Geometry check sheet. Reference: the model listing, model coordinates, mm. Coordinates: 2 decimals unless noted, no trailing zeros. Write each loop counter-clockwise with the first axis right and the second up, starting at its lowest first coordinate (ties: lowest second). Pieces come first, ordered by that corner, then holes. Notation, with made-up numbers: (26, 61) -> (56, 61) arc R15 cw to (56, 65) -> close; hole circle Ø7 at (88, 68). An arc over 180 degrees is marked (long way). Answer as CSV lines item,"result".
```python
from build123d import *

# Parameters (mm, degrees)
SKIZZE1_W                       = 45
SKIZZE1_H                       = 85
AUFSATZ_LINEAR_AUSTRAGEN1_DEPTH = 5
SKIZZE3_W                       = 5
SKIZZE3_H                       = 1.5
SKIZZE3_H_2                     = 1.241942413
SCHNITT_LINEAR_AUSTRAGEN1_DEPTH = 5
SKIZZE4_R                       = 1.6
SCHNITT_LINEAR_AUSTRAGEN2_DEPTH = 5


with BuildPart() as part:
    # Skizze1 → Aufsatz-Linear austragen1 (new body)
    with BuildSketch(Plane.XY):
        with Locations((22.5, 42.5)):
            Rectangle(SKIZZE1_W, SKIZZE1_H)
    extrude(amount=AUFSATZ_LINEAR_AUSTRAGEN1_DEPTH)

    # Skizze3 → Schnitt-Linear austragen1 (cut)
    with BuildSketch(Plane.XY.offset(5)):
        with Locations((12.5, 58.8)):
            Rectangle(SKIZZE3_W, SKIZZE3_H)
        with Locations((32.75, 58.8)):
            Rectangle(SKIZZE3_W, SKIZZE3_H)
        with Locations((19.25, 46.8)):
            Rectangle(SKIZZE3_W, SKIZZE3_H)
        with Locations((12.5, 50.8)):
            Rectangle(SKIZZE3_W, SKIZZE3_H)
        with Locations((32.75, 50.8)):
            Rectangle(SKIZZE3_W, SKIZZE3_H)
        with Locations((12.5, 42.8)):
            Rectangle(SKIZZE3_W, SKIZZE3_H)
        with Locations((32.75, 42.8)):
            Rectangle(SKIZZE3_W, SKIZZE3_H)
        with Locations((12.5, 34.8)):
            Rectangle(SKIZZE3_W, SKIZZE3_H)
        with Locations((32.75, 34.8)):
            Rectangle(SKIZZE3_W, SKIZZE3_H)
        with Locations((32.75, 26.8)):
            Rectangle(SKIZZE3_W, SKIZZE3_H)
        with Locations((12.5, 26.8)):
            Rectangle(SKIZZE3_W, SKIZZE3_H)
        with Locations((19.25, 54.929028794)):
            Rectangle(SKIZZE3_W, SKIZZE3_H_2)
        with Locations((26, 54.929028794)):
            Rectangle(SKIZZE3_W, SKIZZE3_H_2)
        with Locations((26, 46.8)):
            Rectangle(SKIZZE3_W, SKIZZE3_H)
        with Locations((26, 38.8)):
            Rectangle(SKIZZE3_W, SKIZZE3_H)
        with Locations((19.25, 38.8)):
            Rectangle(SKIZZE3_W, SKIZZE3_H)
        with Locations((19.25, 30.8)):
            Rectangle(SKIZZE3_W, SKIZZE3_H)
        with Locations((26, 30.8)):
            Rectangle(SKIZZE3_W, SKIZZE3_H)
        with Locations((26, 22.8)):
            Rectangle(SKIZZE3_W, SKIZZE3_H)
        with Locations((19.25, 22.8)):
            Rectangle(SKIZZE3_W, SKIZZE3_H)
    extrude(amount=-SCHNITT_LINEAR_AUSTRAGEN1_DEPTH, mode=Mode.SUBTRACT)

    # Skizze4 → Schnitt-Linear austragen2 (cut)
    with BuildSketch(Plane.XY.offset(5)):
        with Locations((6, 80)):
            Circle(SKIZZE4_R)
        with Locations((39, 79)):
            Circle(SKIZZE4_R)
        with Locations((39, 5)):
            Circle(SKIZZE4_R)
        with Locations((6, 5)):
            Circle(SKIZZE4_R)
    extrude(amount=-SCHNITT_LINEAR_AUSTRAGEN2_DEPTH, mode=Mode.SUBTRACT)


solid = part.part
```
Item 1: Thickness scan on probe 1 along Y at (x, z) = (11, 2.9); probe 2 along Y at (x, z) = (6, 3.7); probe 3 along Y at (x, z) = (39, 3.9). Record the ranges inside material, lowest first.
Responses:
probe 1,"y = 0 to 26.05, 27.55 to 34.05, 35.55 to 42.05, 43.55 to 50.05, 51.55 to 58.05, 59.55 to 85"
probe 2,"y = 0 to 3.4, 6.6 to 78.4, 81.6 to 85"
probe 3,"y = 0 to 3.4, 6.6 to 77.4, 80.6 to 85"
Item 2: Cross-section at B-B, the plane z = 1.7. Count the separate pieces of the cut face and the enclosed holes in it, plus the area to 3 significant figures.
Responses:
separate pieces,"1"
enclosed holes,"24"
area,"3,650 mm2"
Item 3: Cross-section at A-A, the plane x = 6. Record the cut outline in (y, z).
Responses:
outline,"(0, 0) -> (3.4, 0) -> (3.4, 5) -> (0, 5) -> close; (6.6, 0) -> (78.4, 0) -> (78.4, 5) -> (6.6, 5) -> close; (81.6, 0) -> (85, 0) -> (85, 5) -> (81.6, 5) -> close"
Item 4: Release check for a two-part mould opening along Y. For faces 1 (the flat face through (22, 85, 2)), 2 (the flat face through (12, 26.05, 3)), 3 (the flat face through (22, 43, 5)) record: +Y half, -Y half, draft (parallel to the pull), parting line (faces both ways), or undercut.
Responses:
face 1,"+Y half"
face 2,"undercut"
face 3,"draft"
